The figure shows three views and two pictorial views of one solid part (mm, origin at its lowest corner). Answer the questions. Coordinates: 2 decimals unless noted, no trailing zeros. Loops run counter-clockwise (first coordinate to the right, second up) from the corner with the lowest first, then second, coordinate; pieces in that order, holes last.
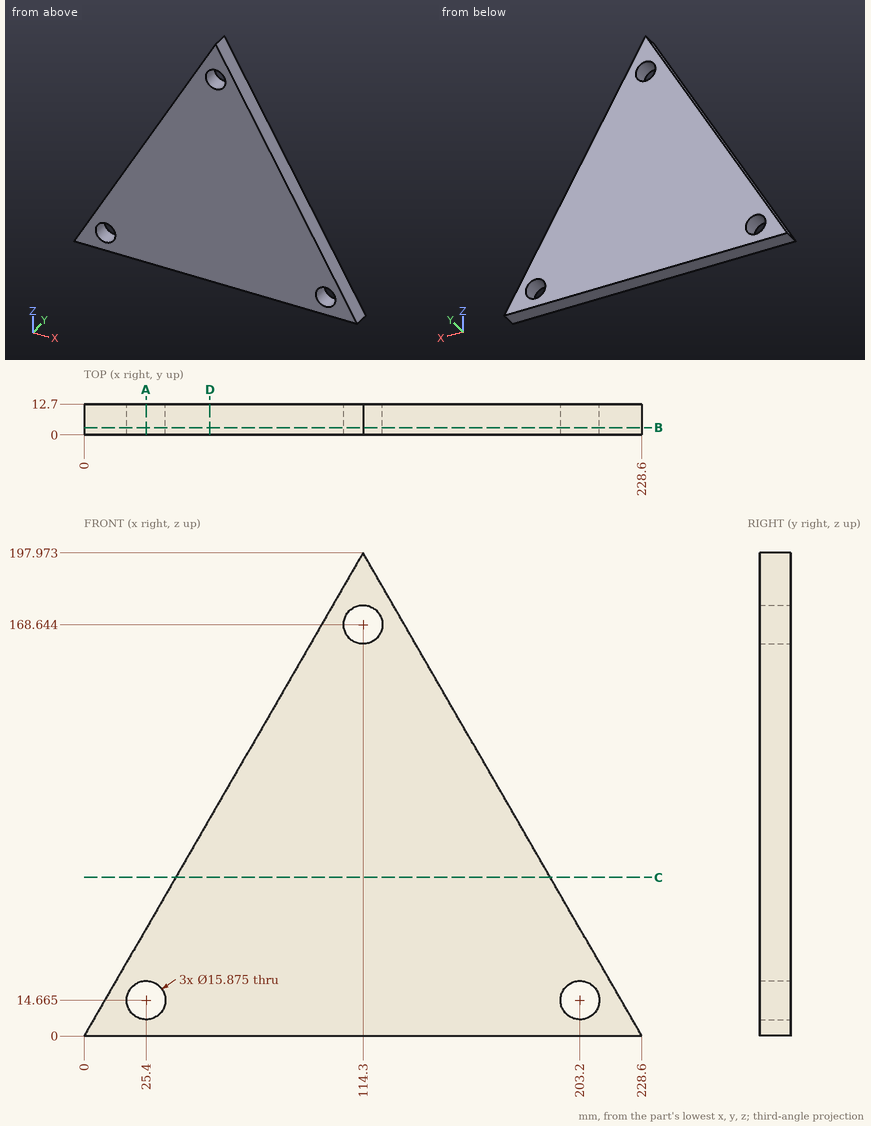
Q1. A cutting plane is placed at B-B (y = 3). Give the vertices of the cut face in (x, z) (1 decimal), then the cut area to 3 significant figures.
Findings below:
outline: (0, 0) - (228.6, 0) - (114.3, 198) - close; hole circle Ø15.9 at (25.4, 14.7); hole circle Ø15.9 at (114.3, 168.6); hole circle Ø15.9 at (203.2, 14.7)
area: 22,000 mm2
Q2. Flat-ended cylindrical pins translate along their axes: pin 1 Ø12.5 at (x, z) = (114.3, 168.64) entering from +Y; pin 2 Ø3 at (y, z) = (1.5, 121) entering from +X; pin 3 Ø1 at (y, z) = (2, 133) entering from -X; pin 4 Ø5 at (x, y) = (112, 10) entering from +Z. Find the tip coordinate at first contact, or state that the pin passes through.
Findings below:
pin 1: passes through
pin 2: stops at x = 159.61
pin 3: stops at x = 76.5
pin 4: stops at z = 197.97
Q3. Straight lines are drawn through the part: probe 1 along Z at (x, y) = (25.4, 2.75) (1 decimal); probe 2 along Z at (x, y) = (198, 2.5) (1 decimal); probe 3 along X at (y, z) = (1.25, 111) (1 decimal). For each, find the intervals that lie inside material, in ascending order.
Findings below:
probe 1: z = 0 to 6.7, 22.6 to 44
probe 2: z = 0 to 8.7, 20.7 to 53
probe 3: x = 64.1 to 164.5
Q4. A cutting plane is placed at A-A (x = 25.4). Give the vertices of the cut face in (y, z).
Findings below:
outline: (0, 0) - (12.7, 0) - (12.7, 6.73) - (0, 6.73) - close; (0, 22.6) - (12.7, 22.6) - (12.7, 43.99) - (0, 43.99) - close
Q5. A cutting plane is placed at D-D (x = 51.5). Give the vertices of the cut face in (y, z), then the cut area to 3 significant figures.
Findings below:
outline: (0, 0) - (12.7, 0) - (12.7, 89.2) - (0, 89.2) - close
area: 1,130 mm2
Q6. A cutting plane is placed at C-C (z = 65). Give the vertices of the cut face in (x, y), then the cut area to 3 significant figures.
Findings below:
outline: (37.53, 0) - (191.07, 0) - (191.07, 12.7) - (37.53, 12.7) - close
area: 1,950 mm2
